from build123d import *

# Parameters (mm, degrees)
SKETCH1_R           = 8.25
BOSS_EXTRUDE1_DEPTH = 5
SKETCH2_R           = 1
CUT_EXTRUDE1_DEPTH  = 2
SKETCH3_R           = 1.75
SKETCH3_R_2         = 0.75
BOSS_EXTRUDE2_DEPTH = 2
SKETCH4_R           = 0.5
BOSS_EXTRUDE3_DEPTH = 2


with BuildPart() as part:
    # Sketch1 → Boss-Extrude1 (new body)
    with BuildSketch(Plane.XY):
        Circle(SKETCH1_R)
    extrude(amount=BOSS_EXTRUDE1_DEPTH)

    # Sketch2 → Cut-Extrude1 (cut)
    with BuildSketch(Plane.XY.offset(5)):
        Circle(SKETCH2_R)
    extrude(amount=-CUT_EXTRUDE1_DEPTH, mode=Mode.SUBTRACT)

    # Sketch3 → Boss-Extrude2 (add)
    with BuildSketch(Plane(origin=(0, 0, 0), x_dir=(-1, 0, 0), z_dir=(0, 0, -1))):
        with Locations(Location((-5.5, 0, 0), (0, 0, 180))):
            Circle(SKETCH3_R)
        with Locations(Location((5.5, 0, 0), (0, 0, 180))):
            Circle(SKETCH3_R)
        with Locations(Location((0, 5.5, 0), (0, 0, 180))):
            Circle(SKETCH3_R_2)
        with Locations(Location((0, -5.5, 0), (0, 0, 180))):
            Circle(SKETCH3_R_2)
    extrude(amount=BOSS_EXTRUDE2_DEPTH)

    # Sketch4 → Boss-Extrude3 (add)
    with BuildSketch(Plane(origin=(0, 0, -2), x_dir=(-1, 0, 0), z_dir=(0, 0, -1))):
        with Locations((-5.5, 0)):
            Circle(SKETCH4_R)
        with Locations((5.5, 0)):
            Circle(SKETCH4_R)
    extrude(amount=BOSS_EXTRUDE3_DEPTH)


solid = part.part
The model under review builds one solid part; all positions refer to its coordinate system, in mm. A direction names the side the tool comes from. Round coordinates to 2 decimals unless told otherwise and drop trailing zeros. Loops run counter-clockwise (first coordinate to the right, second up) from the corner with the lowest first, then second, coordinate; pieces in that order, holes last. Notation, with made-up numbers: (-22.75, -15.5) - (31.25, -15.5) arc R8 cw to (31.25, -3.5) - close; hole circle Ø2 at (74, 17). An arc over 180 degrees is marked (long way). Use CSV: the item, a comma, the result in double quotes.
(1) Clearance check with flat-ended pins moving along their axes: P1, Ø4, axis at x = 3, z = 2.5, coming from the +Y side; P2, Ø5, axis at y = -0.5, z = 0, coming from the +X side; P3, Ø1.2, axis at x = 0, y = 5.5, coming from the -Z side; P4, Ø1, axis at x = 1.5, z = -3, coming from the -Y side. State where each tip first meets the part, or that it passes through.
Working result:
P1,"stops at y = 8.19"
P2,"stops at x = 8.25"
P3,"stops at z = -2"
P4,"passes through"
(2) Take a section at B-B, the plane y = 0. Give the boundary of the cut face in (x, z).
Working result:
outline,"(-8.25, 0) - (-7.25, 0) - (-7.25, -2) - (-6, -2) - (-6, -4) - (-5, -4) - (-5, -2) - (-3.75, -2) - (-3.75, 0) - (3.75, 0) - (3.75, -2) - (5, -2) - (5, -4) - (6, -4) - (6, -2) - (7.25, -2) - (7.25, 0) - (8.25, 0) - (8.25, 5) - (1, 5) - (1, 3) - (-1, 3) - (-1, 5) - (-8.25, 5) - close"
(3) The part is to be moulded in two halves that separate along X. For faces 4 (the cylindrical face through (7.62, -3.16, 2.46)), 5 (the flat face through (0, 5, -2)), 6 (the cylindrical face through (3.75, -0.08, -0.99)), say which applies: pulls with the +X half, pulls with the -X half, needs draft (parallel to the pull), parting line crosses it, or undercut.
Working result:
face 4,"parting line crosses it"
face 5,"needs draft"
face 6,"undercut"
(4) Take a section at C-C, the plane z = 0.25. Give the boundary of the cut face in (x, y).
Working result:
outline,"circle Ø16.5 at (0, 0)"
(5) Machinability: for faces 1 (the cylindrical face through (0, -1, 4)), 2 (the cylindrical face through (6, 0, -3)), 3 (the flat face through (0, -2, 5)), which of the approach directions +Z, -Z, +X, -X, +Y, -Y give a long, thin tool a straight path to every point of the face, cutting with its end or side? Answer none if there is none.
Working result:
face 1,"+Z"
face 2,"-Z"
face 3,"+Z, +X, -X, +Y, -Y"
(6) Take a section at D-D, the plane x = 4.5. Give the boundary of the cut face in (y, z).
Working result:
outline,"(-6.91, 0) - (-1.44, 0) - (-1.44, -2) - (1.44, -2) - (1.44, 0) - (6.91, 0) - (6.91, 5) - (-6.91, 5) - close"
(7) Take a section at A-A, the plane x = 0. Give the boundary of the cut face in (y, z).
Working result:
outline,"(-8.25, 0) - (-6.25, 0) - (-6.25, -2) - (-4.75, -2) - (-4.75, 0) - (4.75, 0) - (4.75, -2) - (6.25, -2) - (6.25, 0) - (8.25, 0) - (8.25, 5) - (1, 5) - (1, 3) - (-1, 3) - (-1, 5) - (-8.25, 5) - close"
(8) For line 1 (Y direction, x = 0, z = 4); line 2 (Z direction, x = 7.75, y = -2); line 3 (Z direction, x = 4.75, y = 1.5), list the stretches that pass through material, from the lowest coordinate up.
Working result:
line 1,"y = -8.25 to -1, 1 to 8.25"
line 2,"z = 0 to 5"
line 3,"z = -2 to 5"
